Geometry check sheet. Reference: drawing and pictorial views, mm from the part's lowest x, y, z. A direction names the side the tool comes from. Give positions to 0.01 mm unless a question says otherwise; leave off trailing zeros. Loops run counter-clockwise (first coordinate to the right, second up) from the corner with the lowest first, then second, coordinate; pieces in that order, holes last. Notation, with made-up numbers: (-21, -0.5) -> (20, -0.5) arc R20 ccw to (20, 3.5) -> close; hole circle Ø7 at (25.5, 29). An arc over 180 degrees is marked (long way). One line per item, written item: value. Start each with the question number.
(1) Sectioned sample at C-C, the plane y = 39. Record the cut outline in (x, z).
(2) Scan lines: line 1 along Y through (x, z) = (7.25, 14.5); line 2 along X through (y, z) = (30.5, 12.25); line 3 along Z through (x, y) = (1.5, 44). Record each from-to range of solid material in increasing order. Write a range as from..to.
(3) Sectioned sample at A-A, the plane x = 12.5. Record the cut outline in (y, z).
(4) Gauge pin test, flat ends, axial feed: pin 1 Ø1.5 at (y, z) = (28, 10.5) entering from -X; pin 2 Ø4 at (x, y) = (10, 45) entering from +Z; pin 3 Ø5 at (y, z) = (45, 19) entering from -X; pin 4 Ø10 at (y, z) = (50, 13.5) entering from +X. Record the tip position at first contact, or that the pin passes through.
(5) Sectioned sample at D-D, the plane x = 22.5. Record the cut outline in (y, z), then the cut area to 3 significant figures.
(6) Tool access check on the marked faces 1 and 2. Record the directions out of +Z, -Z, +X, -X, +Y, -Y that give a thin tool (end or side, any length) a straight path to the whole face; none if there is none.
(7) Sectioned sample at B-B, the plane z = 12.5. Record the cut outline in (x, y).
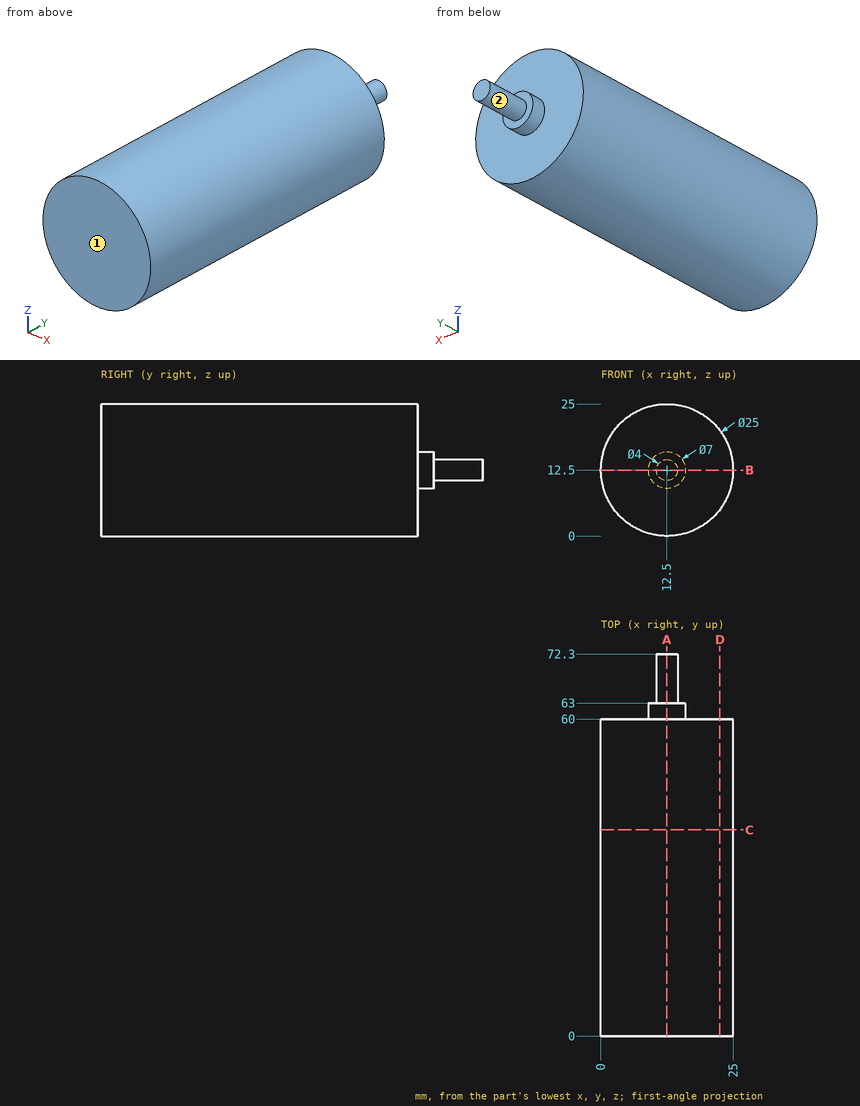
Calculated:
1. outline: circle Ø25 at (12.5, 12.5)
2. line 1: y = 0..60
2. line 2: x = 0..25
2. line 3: z = 6.56..18.44
3. outline: (0, 0) -> (60, 0) -> (60, 9) -> (63, 9) -> (63, 10.5) -> (72.3, 10.5) -> (72.3, 14.5) -> (63, 14.5) -> (63, 16) -> (60, 16) -> (60, 25) -> (0, 25) -> close
4. pin 1: stops at x = 0.06
4. pin 2: stops at z = 24.99
4. pin 3: stops at x = 0.66
4. pin 4: stops at x = 25
5. outline: (0, 5) -> (60, 5) -> (60, 20) -> (0, 20) -> close
5. area: 900 mm2
6. face 1: +Z, -Z, +X, -X, -Y
6. face 2: +Y
7. outline: (0, 0) -> (25, 0) -> (25, 60) -> (16, 60) -> (16, 63) -> (14.5, 63) -> (14.5, 72.3) -> (10.5, 72.3) -> (10.5, 63) -> (9, 63) -> (9, 60) -> (0, 60) -> close
